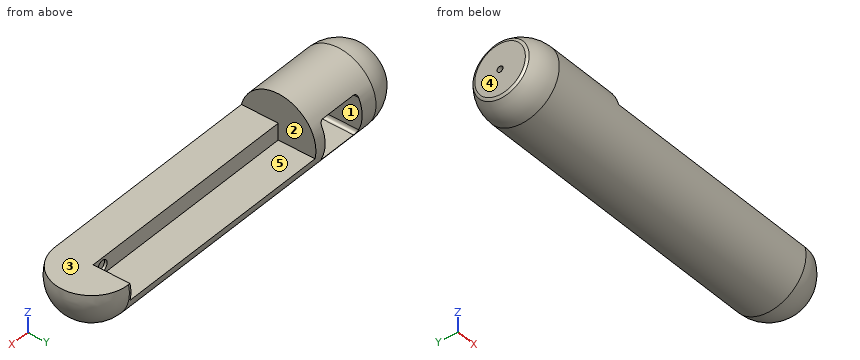
from build123d import *

# Parameters (mm, degrees)
CUT_EXTRUDE7_DEPTH               = 1010.950493836
CUT_EXTRUDE7_DEPTH_BACK          = 1010.950493836
SKETCH13_W                       = 48.176434887
SKETCH13_H                       = 155.804640487
SKETCH4_W                        = 600
SKETCH4_H                        = 44.158972604
CUT_EXTRUDE2_DEPTH               = 1010.950493836
SKETCH7_W                        = 159.807953253
SKETCH7_H                        = 69.49104999
BOSS_EXTRUDE7_DEPTH              = 5
FILLET5_R                        = 10
F_5_8_0_625_DIAMETER_HOLE1_D     = 15.875
F_5_8_0_625_DIAMETER_HOLE1_DEPTH = 30
F_5_8_0_625_DIAMETER_HOLE1_TIP   = 4.769331164
BOSS_EXTRUDE8_DEPTH              = 10
BOSS_EXTRUDE8_DEPTH_BACK         = 10
SKETCH16_W                       = 57.403477863
SKETCH16_H                       = 23.203595883
SKETCH17_W                       = 38.256761469
SKETCH17_H                       = 12.64819079
BOSS_EXTRUDE9_DEPTH              = 10
SKETCH18_W                       = 120
SKETCH18_H                       = 104.74536306
CUT_EXTRUDE8_DEPTH               = 161
FILLET6_R                        = 10
SKETCH19_R                       = 15
CUT_EXTRUDE9_DEPTH               = 7
CUT_EXTRUDE11_DEPTH              = 1010.950493856
CUT_EXTRUDE11_DEPTH_BACK         = 1010.950493856
SKETCH22_W                       = 1481.455902665
SKETCH22_H                       = 524.99926461


# Read off the part's stored shape, not the designer's step: Revolve1
with BuildPart() as part:
    # Revolve1 outline → Revolve1 (revolve)
    with BuildSketch(Plane.YX):
        with BuildLine():
            Line((0, 1000), (0, 0))
            ThreePointArc((0, 0), (70.710678154, 29.289321917), (100, 100.0000001))
            Line((100, 100.0000001), (100, 899.9999999))
            ThreePointArc((100, 899.9999999), (70.710678154, 970.710678083), (0, 1000))
        make_face()
    revolve(axis=Axis((0, 0, 0), (1, 0, 0)))

    # Sketch13 → Cut-Extrude7 (cut, two sides: drawn at the far end of the back side and taken through both)
    with BuildSketch(Plane(origin=(0, 0, 0), x_dir=(1, 0, 0), z_dir=(0, 1, 0)).offset(-CUT_EXTRUDE7_DEPTH_BACK)):
        with Locations((5.911782557, -3.075091589)):
            Rectangle(SKETCH13_W, SKETCH13_H)
    extrude(amount=CUT_EXTRUDE7_DEPTH + CUT_EXTRUDE7_DEPTH_BACK, mode=Mode.SUBTRACT)

    # Sketch4 → Cut-Extrude2 (cut, through all)
    with BuildSketch(Plane(origin=(0, 0, 0), x_dir=(1, 0, 0), z_dir=(0, 1, 0))):
        with Locations((595, 0)):
            Rectangle(SKETCH4_W, SKETCH4_H)
    extrude(amount=CUT_EXTRUDE2_DEPTH, mode=Mode.SUBTRACT)

    # Sketch7 → Boss-Extrude7 (add)
    with BuildSketch(Plane(origin=(0, 0, 0), x_dir=(1, 0, 0), z_dir=(0, 1, 0))):
        with Locations((745.885521462, -1.405844332)):
            Rectangle(SKETCH7_W, SKETCH7_H)
    extrude(amount=-BOSS_EXTRUDE7_DEPTH)

    # Fillet5
    fillet5_edges = [part.edges().sort_by_distance(p)[0] for p in [
        (30, -71.414284286, 0),
    ]]
    fillet(fillet5_edges, radius=FILLET5_R)

    # 5/8 (0.625) Diameter Hole1
    with Locations(Plane.ZY.offset(-30)):
        with Locations((0, 0)):
            Hole(F_5_8_0_625_DIAMETER_HOLE1_D / 2, depth=F_5_8_0_625_DIAMETER_HOLE1_DEPTH)
            with Locations((0, 0, -(F_5_8_0_625_DIAMETER_HOLE1_DEPTH + F_5_8_0_625_DIAMETER_HOLE1_TIP / 2))):  # 118° drill point
                Cone(0, F_5_8_0_625_DIAMETER_HOLE1_D / 2, F_5_8_0_625_DIAMETER_HOLE1_TIP, mode=Mode.SUBTRACT)

    # Sketch16 → Boss-Extrude8 (add, two sides: drawn at the far end of the back side and taken through both)
    with BuildSketch(Plane.XY.offset(-BOSS_EXTRUDE8_DEPTH_BACK)):
        with Locations((738.294537666, -11.601797942)):
            Rectangle(SKETCH16_W, SKETCH16_H)
    extrude(amount=BOSS_EXTRUDE8_DEPTH + BOSS_EXTRUDE8_DEPTH_BACK)

    # Sketch17 → Boss-Extrude9 (add)
    with BuildSketch(Plane.XY.offset(-22.079486302)):
        with Locations((787.071835847, 6.324095395)):
            Rectangle(SKETCH17_W, SKETCH17_H)
    extrude(amount=-BOSS_EXTRUDE9_DEPTH)

    # Sketch18 → Cut-Extrude8 (cut)
    with BuildSketch(Plane(origin=(0, 0, 0), x_dir=(1, 0, 0), z_dir=(0, 1, 0))):
        with Locations((204.992275313, 0)):
            Rectangle(SKETCH18_W, SKETCH18_H)
    extrude(amount=CUT_EXTRUDE8_DEPTH, mode=Mode.SUBTRACT)

    # Fillet6
    fillet6_edges = [part.edges().sort_by_distance(p)[0] for p in [
        (144.992275313, 42.594313674, -52.37268153),
        (144.992275313, 42.594313674, 52.37268153),
        (264.992275313, 42.594313674, 52.37268153),
        (264.992275313, 42.594313674, -52.37268153),
    ]]
    fillet(fillet6_edges, radius=FILLET6_R)

    # Sketch19 → Cut-Extrude9 (cut)
    with BuildSketch(Plane(origin=(0, 0, 0), x_dir=(1, 0, 0), z_dir=(0, 1, 0))):
        with Locations(Location((865, 0, 0), (0, 0, 270))):
            Circle(SKETCH19_R)
    extrude(amount=-CUT_EXTRUDE9_DEPTH, mode=Mode.SUBTRACT)

    # Sketch22 → Cut-Extrude11 (cut, two sides: drawn at the far end of the back side and taken through both)
    with BuildSketch(Plane(origin=(0, 0, 0), x_dir=(1, 0, 0), z_dir=(0, 1, 0)).offset(-CUT_EXTRUDE11_DEPTH_BACK)):
        with Locations((406.155110175, 0)):
            Rectangle(SKETCH22_W, SKETCH22_H)
        Polygon((-101.289974143, 163.942834617), (1092.059469606, 163.942834617), (1092.059469606, -22.079486302), (295, -22.079486302), (295, -179.828704734), (-101.289974143, -179.828704734), (-101.289974143, -22.079486302), align=None, mode=Mode.SUBTRACT)
    extrude(amount=CUT_EXTRUDE11_DEPTH + CUT_EXTRUDE11_DEPTH_BACK, mode=Mode.SUBTRACT)


solid = part.part
Check sheet for the modelled part. Datum: model origin and axes. Units: mm. Face numbers are marked on the shaded views. A direction names the side the tool comes from. Give positions to 0.01 mm unless a question says otherwise; leave off trailing zeros. Write item = value, one per line.
Item 1: Release check for a two-part mould opening along X. For the marked faces 3, 4 and 5 record: +X half, -X half, draft (parallel to the pull), parting line (faces both ways), or undercut.
Output:
face_3 = draft
face_4 = -X half
face_5 = undercut
Item 2: Gauge pin test, flat ends, axial feed: pin 1 (1.5 mm diameter, centred on y = 54, z = 23, fed in from +X); pin 2 (1.5 mm diameter, centred on x = 140, z = 50.5, fed in from -Y); pin 3 (12 mm diameter, centred on x = 670.5, y = 45, fed in from -Z). Record the tip position at first contact, or that the pin passes through.
Output:
pin_1 = 295
pin_2 = -86.75
pin_3 = -92.08
Item 3: Tool access check on the marked faces 1 and 2. Record the directions out of +Z, -Z, +X, -X, +Y, -Y that give a thin tool (end or side, any length) a straight path to the whole face; none if there is none.
Output:
face_1 = +Y
face_2 = +Z, +Y
Item 4: Scan lines: probe 1 along X at (y, z) = (58, -17.5); probe 2 along Z at (x, y) = (431, 74); probe 3 along Z at (x, y) = (51.75, 0). Record each from-to range of solid material in increasing order. Write a range as from..to.
Output:
probe_1 = 30..144.99, 264.99..295, 895..979.56
probe_2 = -67.26..-22.08
probe_3 = -87.59..-7.94, 7.94..87.59
